Part model, mm, in its own coordinate system. A direction names the side the tool comes from. Round coordinates to 2 decimals unless told otherwise and drop trailing zeros. Loops run counter-clockwise (first coordinate to the right, second up) from the corner with the lowest first, then second, coordinate; pieces in that order, holes last. Notation, with made-up numbers: M -32,50.25 L -4,50.25 A20 cw -4,70.25 Z; hole C 17,5.5 d11. An arc over 180 degrees is marked long. Put each result on its own line as item: value. Start each with the question number.
Autodesk Inventor part; units mm, degrees
ref_plane "YZ Plane" through (0, 0, 0) normal (1, 0, 0) x (0, 1, 0)
ref_plane "XZ Plane" through (0, 0, 0) normal (0, 1, 0) x (-1, 0, 0)
ref_plane "XY Plane" through (0, 0, 0) normal (0, 0, 1) x (1, 0, 0)
sketch "Sketch1" plane through (0, 0, 0) normal (0, 0, 1) x (1, 0, 0)
  circle A0 centre (0, 0) radius 361.95
  circle A1 centre (0, 0) radius 393.7
  dimension "d0" = 723.9
  dimension "d1" = 787.4
extrude "Extrusion1" add sketch "Sketch1" along normal blind 326
sketch "Sketch2" plane through (0, 0, 0) normal (0, 0, -1) x (-1, 0, 0)
  circle A0 centre (0, 0) radius 396.875
  circle A1 centre (0, 0) radius 393.7
  dimension "d4" = 793.75
extrude "Extrusion2" add sketch "Sketch2" against normal blind 50.8
sketch "Sketch3" plane through (0, 0, 0) normal (0, 0, -1) x (-1, 0, 0)
  circle A0 centre (0, 0) radius 396.875
  circle A1 centre (0, 0) radius 393.446
  dimension "d7" = 786.892
extrude "Extrusion3" cut sketch "Sketch3" against normal blind 25.4
chamfer "Chamfer1" distance 3.175 angle 45 1 edges at (-393.7, 0, 50.8)
sketch "Sketch4" plane through (0, 0, 326) normal (0, 0, 1) x (1, 0, 0)
  circle A0 centre (0, 0) radius 381
  circle A1 centre (0, 0) radius 393.7
  dimension "d13" = 762
extrude "Extrusion4" add sketch "Sketch4" along normal blind 12.7
fillet "Fillet1" radius 0.7937 2 edges at (-381, 0, 326) (393.446, 0, 25.4)
chamfer "Chamfer2" distance 0.7937 angle 45 1 edges at (-381, 0, 338.7)
equation "\"d10\" = -0.5 * d1 + 0.5 * d4"
properties part number "A1-19027-400-08 HCWI liner - pup" material "Iron, HCWI"
1. Wall check: L1, parallel to Y at x = 0, z = 173; L2, parallel to Y at x = 0, z = 330; L3, parallel to X at y = -2.5, z = 284.5. Give the ranges that are in metal, low to high.
2. Mould opens along X. For faces 4 (the flat face through (336, -139, 326)), 5 (the conical face through (-85.39, 384.53, 53.78)), 6 (the flat face through (-206, 323, 338.7)) say: released by +X, released by -X, zero draft, split by the parting line, or undercut.
3. Drop flat-ended pins along their axis: pin 1 (8 mm diameter, centred on x = -76.5, z = 247, fed in from +Y); pin 2 (1.5 mm diameter, centred on x = 201.5, z = 59.5, fed in from -Y); pin 3 (6 mm diameter, centred on x = -118, z = 220, fed in from -Y). Give the stop position or say it passes through.
4. Which spindle directions (+Z, -Z, +X, -X, +Y, -Y) get a long thin tool onto all of the face, cutting with end or side? Do faces 1 (the cylindrical face through (375.52, -118.26, 194.34)), 2 (the flat face through (-319, -173, 0)), 3 (the cylindrical face through (85.29, -384.09, 12.13)). Say none if no direction does.
5. Cut at C-C, the plane z = 269.5. Give the cut face in (x, y).
Results list:
1. L1: y = -393.7 to -361.95, 361.95 to 393.7
1. L2: y = -393.7 to -381, 381 to 393.7
1. L3: x = -393.69 to -361.94, 361.94 to 393.69
2. face 4: undercut
2. face 5: split by the parting line
2. face 6: zero draft
3. pin 1: stops at y = 386.97
3. pin 2: stops at y = -338.67
3. pin 3: stops at y = -376.53
4. face 1: +Z
4. face 2: -Z, +X, -X, +Y, -Y
4. face 3: -Z
5. outline: C 0,0 d787.4; hole C 0,0 d723.9
